Read the model definition and answer for the solid it produces. Units are mm, in the model's axes. A direction names the side the tool comes from. Round coordinates to 2 decimals unless told otherwise and drop trailing zeros. Loops run counter-clockwise (first coordinate to the right, second up) from the corner with the lowest first, then second, coordinate; pieces in that order, holes last. Notation, with made-up numbers: (79.25, 63.5) -> (119.25, 63.5) arc R13 ccw to (119.25, 79.5) -> close; hole circle Ø9 at (-9.75, 85). An arc over 180 degrees is marked (long way). Put each result on its own line as item: value.
from build123d import *

# Parameters (mm, degrees)
SKETCH1_W                            = 304.8
SKETCH1_H                            = 127
BOSS_EXTRUDE1_DEPTH                  = 4.7625
SKETCH2_W                            = 25.4
SKETCH2_H                            = 3.175
BOSS_EXTRUDE2_DEPTH                  = 31.115
CUT_EXTRUDE1_DEPTH                   = 63.5
FILLET1_R                            = 5.08
FILLET2_R                            = 12.7
FILLET4_R                            = 6.35
CUT_EXTRUDE2_DEPTH                   = 4.7625
LPATTERN2_COUNT                      = 2
LPATTERN2_PITCH                      = 279.4
LPATTERN2_COUNT_DIR2                 = 2
LPATTERN2_PITCH_DIR2                 = 69.85
SKETCH8_W                            = 25.4
SKETCH8_H                            = 12.7
SKETCH8_H_2                          = 4.6355
BOSS_EXTRUDE3_DEPTH                  = 25.4
CUT_EXTRUDE3_REACH                   = 86.087
SKETCH9_R                            = 3.302
F_13_64_0_20313_DIAMETER_HOLE1_D     = 5.159502
F_13_64_0_20313_DIAMETER_HOLE1_DEPTH = 9.0678
F_13_64_0_20313_DIAMETER_HOLE1_TIP   = 1.550070783
FILLET5_R                            = 6.35
FILLET6_R                            = 3.175
FILLET7_R                            = 1.5875
FILLET11_R                           = 6.35


with BuildPart() as part:
    # Sketch1 → Boss-Extrude1 (new body)
    with BuildSketch(Plane.XY):
        Rectangle(SKETCH1_W, SKETCH1_H)
    extrude(amount=BOSS_EXTRUDE1_DEPTH)

    # Sketch2 → Boss-Extrude2 (add)
    with BuildSketch(Plane(origin=(0, 0, 0), x_dir=(-1, 0, 0), z_dir=(0, 0, -1))):
        with Locations((0, 53.975)):
            Rectangle(SKETCH2_W, SKETCH2_H)
        with Locations((0, -53.975)):
            Rectangle(SKETCH2_W, SKETCH2_H)
    extrude(amount=BOSS_EXTRUDE2_DEPTH)

    # Sketch3 → Cut-Extrude1 (cut, symmetric)
    with BuildSketch(Plane(origin=(0, 0, 0), x_dir=(1, 0, 0), z_dir=(0, 1, 0))):
        with BuildLine():
            Line((2.38125, 26.3525), (2.38125, 31.115))
            Line((2.38125, 31.115), (-2.38125, 31.115))
            Line((-2.38125, 31.115), (-2.38125, 26.3525))
            ThreePointArc((-2.38125, 26.3525), (0, 23.97125), (2.38125, 26.3525))
        make_face()
    extrude(amount=CUT_EXTRUDE1_DEPTH, both=True, mode=Mode.SUBTRACT)

    # Fillet1
    fillet1_edges = [part.edges().sort_by_distance(p)[0] for p in [
        (-2.38125, -53.975, -31.115),
        (2.38125, -53.975, -31.115),
        (-2.38125, 53.975, -31.115),
        (2.38125, 53.975, -31.115),
        (12.7, -53.975, -31.115),
        (-12.7, -53.975, -31.115),
        (-12.7, 53.975, -31.115),
        (12.7, 53.975, -31.115),
    ]]
    fillet(fillet1_edges, radius=FILLET1_R)

    # Fillet2
    fillet2_edges = [part.edges().sort_by_distance(p)[0] for p in [
        (-152.4, 63.5, 2.38125),
        (152.4, 63.5, 2.38125),
        (152.4, -63.5, 2.38125),
        (-152.4, -63.5, 2.38125),
    ]]
    fillet(fillet2_edges, radius=FILLET2_R)

    # Fillet4
    fillet4_edges = [part.edges().sort_by_distance(p)[0] for p in [
        (12.7, 53.975, 0),
        (0, 52.3875, 0),
        (-12.7, 53.975, 0),
        (0, 55.5625, 0),
        (0, -52.3875, 0),
        (12.7, -53.975, 0),
        (0, -55.5625, 0),
        (-12.7, -53.975, 0),
    ]]
    fillet(fillet4_edges, radius=FILLET4_R)

    # Sketch7 → Cut-Extrude2 (cut)
    with BuildSketch(Plane(origin=(0, 0, 0), x_dir=(-1, 0, 0), z_dir=(0, 0, -1))):
        with BuildLine():
            Line((-146.05, 37.1475), (-133.35, 37.1475))
            ThreePointArc((-133.35, 37.1475), (-131.1275, 34.925), (-133.35, 32.7025))
            Line((-133.35, 32.7025), (-146.05, 32.7025))
            ThreePointArc((-146.05, 32.7025), (-148.2725, 34.925), (-146.05, 37.1475))
        make_face()
    cut_extrude2 = extrude(amount=-CUT_EXTRUDE2_DEPTH, mode=Mode.SUBTRACT)

    # LPattern2: Cut-Extrude2 2 × 2
    with Locations(*[(-i * LPATTERN2_PITCH, -j * LPATTERN2_PITCH_DIR2, 0) for i in range(LPATTERN2_COUNT) for j in range(LPATTERN2_COUNT_DIR2) if (i, j) != (0, 0)]):
        add(cut_extrude2, mode=Mode.SUBTRACT)

    # Sketch8 → Boss-Extrude3 (add)
    with BuildSketch(Plane.XY.offset(4.7625)):
        with Locations((0, -22.19325)):
            Rectangle(SKETCH8_W, SKETCH8_H)
        with Locations((0, 18.26895)):
            Rectangle(SKETCH8_W, SKETCH8_H_2)
    extrude(amount=BOSS_EXTRUDE3_DEPTH)

    # Sketch9 → Cut-Extrude3 (cut, up to next)
    with BuildSketch(Plane(origin=(0, 20.5867, 0), x_dir=(1, 0, 0), z_dir=(0, 1, 0)), mode=Mode.PRIVATE) as cut_extrude3_sk1:
        with Locations(Location((-1.812874351, -21.2725, 0), (0, 0, 270))):  # turned: the seam where the file's is
            Circle(SKETCH9_R)
    cut_extrude3_tool1 = extrude(cut_extrude3_sk1.sketch, amount=-CUT_EXTRUDE3_REACH, mode=Mode.PRIVATE) & part.part
    add(cut_extrude3_tool1.solids().sort_by_distance((-1.812874, 20.5867, 21.2725))[0], mode=Mode.SUBTRACT)

    # 13/64 (0.20313) Diameter Hole1
    with Locations(Plane(origin=(0, -15.84325, 0), x_dir=(-1, 0, 0), z_dir=(0, 1, 0))):
        with Locations((1.812886138, 21.2725)):
            Hole(F_13_64_0_20313_DIAMETER_HOLE1_D / 2, depth=F_13_64_0_20313_DIAMETER_HOLE1_DEPTH)
            with Locations((0, 0, -(F_13_64_0_20313_DIAMETER_HOLE1_DEPTH + F_13_64_0_20313_DIAMETER_HOLE1_TIP / 2))):  # 118° drill point
                Cone(0, F_13_64_0_20313_DIAMETER_HOLE1_D / 2, F_13_64_0_20313_DIAMETER_HOLE1_TIP, mode=Mode.SUBTRACT)

    # Fillet5
    fillet5_edges = [part.edges().sort_by_distance(p)[0] for p in [
        (-12.7, -22.19325, 4.7625),
        (12.7, -22.19325, 4.7625),
        (-12.7, 18.26895, 4.7625),
        (12.7, 18.26895, 4.7625),
    ]]
    fillet(fillet5_edges, radius=FILLET5_R)

    # Fillet6
    fillet6_edges = [part.edges().sort_by_distance(p)[0] for p in [
        (-12.7, -22.19325, 30.1625),
        (12.7, -22.19325, 30.1625),
        (-12.7, 18.26895, 30.1625),
        (12.7, 18.26895, 30.1625),
    ]]
    fillet(fillet6_edges, radius=FILLET6_R)

    # Fillet7
    fillet7_edges = [part.edges().sort_by_distance(p)[0] for p in [
        (0, -15.84325, 4.7625),
        (0, 15.9512, 4.7625),
    ]]
    fillet(fillet7_edges, radius=FILLET7_R)

    # Fillet11
    fillet11_edges = [part.edges().sort_by_distance(p)[0] for p in [
        (0, -28.54325, 4.7625),
        (0, 20.5867, 4.7625),
    ]]
    fillet(fillet11_edges, radius=FILLET11_R)


solid = part.part
Item 1: Find the intervals of material crossed by line 1 along Z through (x, y) = (57.5, -47); line 2 along Y through (x, z) = (-4, 9.5); line 3 along Z through (x, y) = (-8.5, -55.5), in increasing order.
Derived:
line 1: z = 0 to 4.76
line 2: y = -28.75 to -15.84, 15.95 to 20.79
line 3: z = -31.04 to 4.76
Item 2: For a pull along Y with two mould halves and no side action, classify faces 1 (the conical face through (-1.716, -26.192, 20.835)), 2 (the flat face through (0, -15.843, 18)), 3 (the cylindrical face through (-0.267, -30.453, 6.573)) as pulls with the +Y half, pulls with the -Y half, needs draft (parallel to the pull), parting line crosses it, or undercut.
Derived:
face 1: pulls with the +Y half
face 2: undercut
face 3: pulls with the -Y half
Item 3: Which of the six approach directions +Z, -Z, +X, -X, +Y, -Y give full straight-line access (tool end or side, diameter ignored) to faces 4 (the flat face through (0, 55.562, -19)), 5 (the flat face through (-12.7, -22, 19)), 6 (the cylindrical face through (-0.622, -20.441, 18.984)), 7 (the flat face through (12.7, -22, 19)), 8 (the flat face through (0, -28.543, 21))?
Derived:
face 4: -Z, +X, -X, +Y
face 5: +Z, -X, +Y, -Y
face 6: +Y
face 7: +Z, +X, +Y, -Y
face 8: +Z, +X, -X, -Y
Item 4: The part is cut by section B-B (y = 4). Determine the outline of the cut face in (x, z), then the cut area to 3 significant figures.
Derived:
outline: (-152.4, 0) -> (152.4, 0) -> (152.4, 4.76) -> (-152.4, 4.76) -> close
area: 1,450 mm^2
Item 5: The part is cut by section A-A (x = 29). Determine the outline of the cut face in (y, z), then the cut area to 3 significant figures.
Derived:
outline: (-63.5, 0) -> (63.5, 0) -> (63.5, 4.76) -> (-63.5, 4.76) -> close
area: 605 mm^2
Item 6: Flat-ended cylindrical pins translate along their axes: pin 1 Ø10 at (x, y) = (-71, -44) entering from +Z; pin 2 Ø5 at (x, z) = (-141.5, 1.5) entering from -Y; pin 3 Ø5 at (y, z) = (17, 16.5) entering from -X; pin 4 Ø4 at (x, z) = (39, 8.5) entering from +Y. Find the tip coordinate at first contact, or state that the pin passes through.
Derived:
pin 1: stops at z = 4.76
pin 2: stops at y = -63.5
pin 3: stops at x = -12.7
pin 4: passes through
